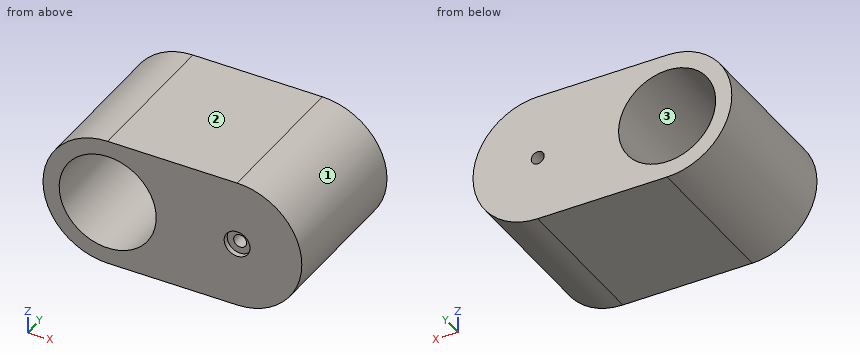
from build123d import *

# Parameters (mm, degrees)
SKETCH3_R           = 22.5
BOSS_EXTRUDE1_DEPTH = 70
SKETCH4_R           = 6
CUT_EXTRUDE1_DEPTH  = 2.5
SKETCH6_R           = 3
CUT_EXTRUDE2_DEPTH  = 6
SKETCH7_R           = 3
CUT_EXTRUDE3_DEPTH  = 118.898261226


with BuildPart() as part:
    # Sketch3 → Boss-Extrude1 (new body)
    with BuildSketch(Plane(origin=(0, 0, 0), x_dir=(1, 0, 0), z_dir=(0, 1, 0))):
        with BuildLine():
            Line((0, 30), (60, 30))
            ThreePointArc((60, 30), (90, 0), (60, -30))
            Line((60, -30), (0, -30))
            ThreePointArc((0, -30), (-30, 0), (0, 30))
        make_face()
        with Locations(Location((0, 0, 0), (0, 0, 270))):
            Circle(SKETCH3_R, mode=Mode.SUBTRACT)
    extrude(amount=BOSS_EXTRUDE1_DEPTH)

    # Sketch4 → Cut-Extrude1 (cut)
    with BuildSketch(Plane.XZ):
        with Locations(Location((60, 0, 0), (0, 0, 270))):
            Circle(SKETCH4_R)
    extrude(amount=-CUT_EXTRUDE1_DEPTH, mode=Mode.SUBTRACT)

    # Sketch6 → Cut-Extrude2 (cut)
    with BuildSketch(Plane.XZ):
        with Locations(Location((60, 0, 0), (0, 0, 270))):
            Circle(SKETCH6_R)
    extrude(amount=-CUT_EXTRUDE2_DEPTH, mode=Mode.SUBTRACT)

    # Sketch7 → Cut-Extrude3 (cut, through all)
    with BuildSketch(Plane(origin=(0, 70, 0), x_dir=(1, 0, 0), z_dir=(0, 1, 0))):
        with Locations(Location((60, 0, 0), (0, 0, 90))):
            Circle(SKETCH7_R)
    extrude(amount=-CUT_EXTRUDE3_DEPTH, mode=Mode.SUBTRACT)


solid = part.part
Part model, mm, in its own coordinate system. Face numbers are marked on the shaded views. Give positions to 0.01 mm unless a question says otherwise; leave off trailing zeros. Loops run counter-clockwise (first coordinate to the right, second up) from the corner with the lowest first, then second, coordinate; pieces in that order, holes last.
(1) Pin check, flat tips, straight feed: pin 1 (12 mm diameter, centred on y = 16, z = 11.5, fed in from +X); pin 2 (1 mm diameter, centred on y = 36, z = 5, fed in from -X); pin 3 (11 mm diameter, centred on x = 60, z = 0, fed in from -Y); pin 4 (3.5 mm diameter, centred on x = 59, z = 0, fed in from -Y). Stop position of each tip, or through.
Return value:
pin 1: stops at x = 89.49
pin 2: stops at x = -29.66
pin 3: stops at y = 2.5
pin 4: passes through
(2) Band-saw the part on A-A (z = 0). Write the cut outline in (x, y).
Return value:
outline: (-30, 0) - (-22.5, 0) - (-22.5, 70) - (-30, 70) - close; (22.5, 0) - (54, 0) - (54, 2.5) - (57, 2.5) - (57, 70) - (22.5, 70) - close; (63, 2.5) - (66, 2.5) - (66, 0) - (90, 0) - (90, 70) - (63, 70) - close
(3) Band-saw the part on C-C (z = -21). Write the cut outline in (x, y).
Return value:
outline: (-21.42, 0) - (-8.08, 0) - (-8.08, 70) - (-21.42, 70) - close; (8.08, 0) - (81.42, 0) - (81.42, 70) - (8.08, 70) - close
(4) Drill centre lines: line 1 along X through (y, z) = (33, 0); line 2 along X through (y, z) = (0.5, 0); line 3 along Z through (x, y) = (60, 31.5). Where is each one in solid material? Low to high.
Return value:
line 1: x = -30 to -22.5, 22.5 to 57, 63 to 90
line 2: x = -30 to -22.5, 22.5 to 54, 66 to 90
line 3: z = -30 to -3, 3 to 30
(5) Band-saw the part on B-B (x = -6). Write the cut outline in (y, z), and give its area (3 significant figures).
Return value:
outline: (0, -29.39) - (70, -29.39) - (70, -21.69) - (0, -21.69) - close; (0, 21.69) - (70, 21.69) - (70, 29.39) - (0, 29.39) - close
area: 1,080 mm2
(6) Band-saw the part on D-D (y = 17). Write the cut outline in (x, z), and give its area (3 significant figures).
Return value:
outline: (0, -30) - (60, -30) arc R30 ccw to (60, 30) - (0, 30) arc R30 ccw to start; hole circle Ø45 at (0, 0); hole circle Ø6 at (60, 0)
area: 4,810 mm2
(7) Pull direction Z, two halves, no side cores. Call the marked faces 1, 2 and 3: pulls with the +Z half, pulls with the -Z half, needs draft (parallel to the pull), parting line crosses it, or undercut.
Return value:
face 1: parting line crosses it
face 2: pulls with the +Z half
face 3: undercut
